Design review of the part built by this model. Coordinates are the model's own, in mm. A direction names the side the tool comes from. Coordinates: 2 decimals unless noted, no trailing zeros. Loops run counter-clockwise (first coordinate to the right, second up) from the corner with the lowest first, then second, coordinate; pieces in that order, holes last. Notation, with made-up numbers: (-35, 77.5) -> (19, 77.5) arc R20 cw to (19, 85.5) -> close; hole circle Ø3 at (-29.5, 78.25). An arc over 180 degrees is marked (long way). Use a Markdown table: item, result. Add a question column.
Q1. For faces 4 (the face through (-81.74, -52, 3)), 5 (the face through (-18.24, -33, 3)), 6 (the face through (-79, -0.05, 3)), 7 (the face through (-34, -33.07, 3)), list the 3-axis set-ups (+Z, -Z, +X, -X, +Y, -Y) from which the entire face can be reached by the end or side of a thin tool; tool diameter is ignored.
Q2. Draft analysis for pull direction Y (two halves, no side actions). For faces 1 (the face through (-81.74, 13, 3)), 2 (the face through (89.544, 15.077, 3.131)), 3 (the face through (46, -0.05, 3)), state which applies: pulls with the +Y half, pulls with the -Y half, needs draft (parallel to the pull), parting line crosses it, or undercut.
Q3. Take a section at B-B on z = 3. Write out the cut boundary in (x, y).
Q4. Clearance check with flat-ended pins moving along their axes: pin 1 Ø3 at (y, z) = (-19.5, 4) entering from -X; pin 2 Ø6.5 at (x, y) = (87.17, 15.82) entering from -Z; pin 3 Ø2 at (x, z) = (64.5, 3.5) entering from -Y. State where each tip first meets the part, or that it passes through.
Q5. Take a section at C-C on y = -58.5. Write out the cut boundary in (x, z).
Q6. Take a section at A-A on x = -1. Write out the cut boundary in (y, z), plus the area to 3 significant figures.
Q7. For probe 1 along X at (y, z) = (-5, 3.5); probe 2 along Y at (x, z) = (-3, 3.25); probe 3 along X at (y, z) = (17, 1.75), list the stretches that pass through material, from the lowest coordinate up.
Q8. Take a section at D-D on x = 48. Write out the cut boundary in (y, z).
Autodesk Inventor part; units mm, degrees
ref_plane "YZ Plane" through (0, 0, 0) normal (1, 0, 0) x (0, 1, 0)
ref_plane "XZ Plane" through (0, 0, 0) normal (0, 1, 0) x (-1, 0, 0)
ref_plane "XY Plane" through (0, 0, 0) normal (0, 0, 1) x (1, 0, 0)
sketch "Sketch2" plane through (0, 0, 0) normal (0, 0, 1) x (1, 0, 0)
  line L0 (-75.3899, 25.3495) -> (108.7601, 25.3495)
  line L1 (108.7601, 25.3495) -> (108.7601, -0.0505)
  line L2 (108.7601, -0.0505) -> (-18.2399, -0.0505)
  line L3 (-75.3899, 25.3495) -> (-75.3899, -64.8205)
  line L4 (-75.3899, -64.8205) -> (-18.2399, -64.8205)
  line L5 (-18.2399, -64.8205) -> (-18.2399, -0.0505)
  line L6 (-75.3899, 25.3495) -> (-81.7399, 25.3495)
  line L7 (-81.7399, 25.3495) -> (-81.7399, -0.0505)
  line L8 (-81.7399, -0.0505) -> (-75.3899, -0.0505)
  line L9 (-75.3899, -64.8205) -> (-81.7399, -64.8205)
  line L10 (-81.7399, -64.8205) -> (-81.7399, -39.4205)
  line L11 (-81.7399, -39.4205) -> (-75.3899, -39.4205)
  line L12 (108.7601, 25.3495) -> (87.1701, 25.3495)
  line L13 (87.1701, 25.3495) -> (87.1701, 15.8245)
  line L14 (87.1701, 15.8245) -> (36.3701, 15.8245)
  circle A0 centre (36.3701, 15.8245) radius 2.4892
  circle A1 centre (87.1701, 15.8245) radius 2.4892
  line L15 (-18.2399, -64.8205) -> (-18.2399, -45.7705)
  line L16 (-18.2399, -45.7705) -> (-37.2899, -45.7705)
  line L17 (-37.2899, -45.7705) -> (-37.2899, -33.0705)
  line L18 (-37.2899, -33.0705) -> (-30.9399, -33.0705)
  line L19 (-30.9399, -33.0705) -> (-30.9399, -7.6705)
  line L20 (-30.9399, -7.6705) -> (-37.2899, -7.6705)
  line L21 (-37.2899, -7.6705) -> (-37.2899, 5.0295)
  line L22 (-37.2899, 5.0295) -> (-30.9399, 5.0295)
  line L23 (-30.9399, 5.0295) -> (-30.9399, -7.6705)
  line L24 (-30.9399, -33.0705) -> (-30.9399, -45.7705)
  point P0 (0, 0)
  dimension "d5" = 184.15
  dimension "d6" = 25.4
  dimension "d7" = 127
  dimension "d8" = 90.17
  dimension "d9" = 6.35
  dimension "d10" = 25.4
  dimension "d11" = 25.4
  dimension "d12" = 21.59
  dimension "d13" = 9.525
  dimension "d14" = 50.8
  dimension "d15" = 4.9784
  dimension "d16" = 4.9784
  dimension "d17" = 19.05
  dimension "d18" = 19.05
  dimension "d19" = 12.7
  dimension "d20" = 6.35
  dimension "d21" = 25.4
  dimension "d22" = 6.35
  dimension "d23" = 12.7
extrude "Extrusion1" add sketch "Sketch2" along normal blind 6.35
sketch "Sketch3" plane through (0, 0, 6.35) normal (0, 0, 1) x (1, 0, 0)
  line L0 (-81.7399, 25.3495) -> (108.7601, 25.3495)
  line L1 (108.7601, 25.3495) -> (2.0801, 25.3495)
  line L2 (2.0801, 25.3495) -> (2.0801, 15.8245)
  line L3 (2.0801, 15.8245) -> (-10.6199, 15.8245)
  line L4 (-10.6199, 15.8245) -> (-10.6199, 9.4745)
  line L5 (-10.6199, 9.4745) -> (2.0801, 9.4745)
  line L6 (2.0801, 9.4745) -> (2.0801, 15.8245)
  point P0 (0, 0)
  dimension "d26" = 106.68
  dimension "d27" = 9.525
  dimension "d28" = 12.7
  dimension "d29" = 6.35
extrude "Extrusion2" cut sketch "Sketch3" against normal blind 25.4
properties part number "side 1"
Answer list:
| question | item | result |
|---|---|---|
| 1 | face 4 | +Z, -Z, -X, +Y, -Y |
| 1 | face 5 | +Z, -Z, +X, -Y |
| 1 | face 6 | +Z, -Z, -X |
| 1 | face 7 | +Z, -Z |
| 2 | face 1 | needs draft |
| 2 | face 2 | undercut |
| 2 | face 3 | pulls with the -Y half |
| 3 | outline | (-81.74, -64.82) -> (-18.24, -64.82) -> (-18.24, -0.05) -> (108.76, -0.05) -> (108.76, 25.35) -> (-81.74, 25.35) -> (-81.74, -0.05) -> (-75.39, -0.05) -> (-75.39, -39.42) -> (-81.74, -39.42) -> close; hole (-37.29, -45.77) -> (-30.94, -45.77) -> (-30.94, -33.07) -> (-37.29, -33.07) -> close; hole (-37.29, -7.67) -> (-30.94, -7.67) -> (-30.94, 5.03) -> (-37.29, 5.03) -> close; hole (-10.62, 9.47) -> (2.08, 9.47) -> (2.08, 15.82) -> (-10.62, 15.82) -> close; hole circle Ø4.98 at (36.37, 15.82); hole circle Ø4.98 at (87.17, 15.82) |
| 4 | pin 1 | x = -75.39 |
| 4 | pin 2 | z = 0 |
| 4 | pin 3 | y = -0.05 |
| 5 | outline | (-81.74, 0) -> (-18.24, 0) -> (-18.24, 6.35) -> (-81.74, 6.35) -> close |
| 6 | outline | (-0.05, 0) -> (9.47, 0) -> (9.47, 6.35) -> (-0.05, 6.35) -> close; (15.82, 0) -> (25.35, 0) -> (25.35, 6.35) -> (15.82, 6.35) -> close |
| 6 | area | 121 mm² |
| 7 | probe 1 | -75.39 to -37.29, -30.94 to -18.24 |
| 7 | probe 2 | -0.05 to 9.47, 15.82 to 25.35 |
| 7 | probe 3 | -81.74 to 34.18, 38.56 to 84.98, 89.36 to 108.76 |
| 8 | outline | (-0.05, 0) -> (25.35, 0) -> (25.35, 6.35) -> (-0.05, 6.35) -> close |
